Verification items for the finished model (mm, model axes). A direction names the side the tool comes from. Round coordinates to 2 decimals unless told otherwise and drop trailing zeros. Write each loop counter-clockwise with the first axis right and the second up, starting at its lowest first coordinate (ties: lowest second). Pieces come first, ordered by that corner, then holes. Notation, with made-up numbers: M 69.5,-14 L 114.5,-14 A3 cw 114.5,-9 Z; hole C -29,-22 d7. An arc over 180 degrees is marked long. Use a Markdown table: item, result. Add a question column.
from build123d import *

# Parameters (mm, degrees)
F0_W     = 58
F0_H     = 137.16
F0_R     = 1.524
F1_DEPTH = 1.27
F2_START = 1.27
F2_DEPTH = 24.13


with BuildPart() as f1:
    # F0 (on Top) → F1 (new body)
    with BuildSketch(Plane.XY):
        with Locations((0, -52.8447)):
            Rectangle(F0_W, F0_H)
        with BuildLine():
            Line((-29, 15.7353), (29, 15.7353))
            Line((29, 15.7353), (29, 21.4803))
            ThreePointArc((29, 21.4803), (28.0700640303, 23.7253640303), (25.825, 24.6553))
            Line((25.825, 24.6553), (-25.825, 24.6553))
            ThreePointArc((-25.825, 24.6553), (-28.0700640303, 23.7253640303), (-29, 21.4803))
            Line((-29, 21.4803), (-29, 15.7353))
        make_face()
        with Locations((-26.1366, 21.7678)):
            Circle(F0_R, mode=Mode.SUBTRACT)
        with Locations((26.1366, 21.7678)):
            Circle(F0_R, mode=Mode.SUBTRACT)
        with BuildLine():
            Line((-25.825, -130.3447), (25.825, -130.3447))
            ThreePointArc((25.825, -130.3447), (28.0700640303, -129.4147640303), (29, -127.1697))
            Line((29, -127.1697), (29, -121.4247))
            Line((29, -121.4247), (-29, -121.4247))
            Line((-29, -121.4247), (-29, -127.1697))
            ThreePointArc((-29, -127.1697), (-28.0700640303, -129.4147640303), (-25.825, -130.3447))
        make_face()
        with Locations((-26.1366, -127.4572)):
            Circle(F0_R, mode=Mode.SUBTRACT)
        with Locations((26.1366, -127.4572)):
            Circle(F0_R, mode=Mode.SUBTRACT)
    extrude(amount=F1_DEPTH)

    # F0 (on Top) → F2 (join)
    with BuildSketch(Plane.XY.offset(F2_START)):
        with Locations((0, -52.8447)):
            Rectangle(F0_W, F0_H)
    extrude(amount=F2_DEPTH)

    # F3 (on Right) → F4 (revolve)
    with BuildSketch(Plane.YZ):
        Polygon((5.8928, 70.612), (3.4461211403, 70.612), (2, 68.199), (0, 68.199), (0, 25.4), (14.2875, 25.4), (14.2875, 53.2638), (5.8928, 69.85), align=None)
    revolve(axis=Axis((0, 0, 43.7137000263), (0, 0, 1)))


solid = f1.part
1. Release check for a two-part mould opening along Y. For faces 4 (the flat face through (0, 0, 68.199)), 5 (the cylindrical face through (-0.628, -14.274, 39.527)), 6 (the flat face through (0, -52, 0)), 7 (the cylindrical face through (-28.045, 23.75, 0.626)) record: +Y half, -Y half, draft (parallel to the pull), parting line (faces both ways), or undercut.
2. Cross-section at C-C on z = 18. Enter the section's corners in (x, y).
3. Scan lines: line 1 along Z through (x, y) = (17.5, -103); line 2 along Y through (x, z) = (1, 46.5); line 3 along Y through (x, z) = (3, 7). Record each from-to range of solid material in increasing order. Write a range as from..to.
4. Access from +Z, -Z, +X, -X, +Y, -Y to the whole of each face (thin tool, end or side, straight path). Record for faces 1 (the flat face through (0, 15.735, 13)), 2 (the cylindrical face through (-1.77, 5.62, 70.24)), 3 (the flat face through (0, -126, 1.27)).
5. Cross-section at D-D on x = 0. Enter the section's corners in (y, z).
6. Cross-section at B-B on y = 0. Enter the section's corners in (x, z), plus the area to 3 significant figures.
7. Cross-section at A-A on x = 17. Enter the section's corners in (y, z), plus the area to 3 significant figures.
8. Depth check by flat-ended pin: pin 1 Ø4.5 at (x, y) = (7.5, 19) entering from +Z; pin 2 Ø8 at (x, z) = (-4.5, 53.5) entering from -Y; pin 3 Ø7 at (x, z) = (6.5, 9) entering from +Y. Enter the tip coordinate at first touch or a pass-through.
Answer:
| question | item | result |
|---|---|---|
| 1 | face 4 | undercut |
| 1 | face 5 | parting line |
| 1 | face 6 | draft |
| 1 | face 7 | +Y half |
| 2 | outline | M -29,-121.42 L 29,-121.42 L 29,15.74 L -29,15.74 Z |
| 3 | line 1 | z = 0..25.4 |
| 3 | line 2 | y = -14.25..14.25 |
| 3 | line 3 | y = -121.42..15.74 |
| 4 | face 1 | +Z, +X, -X, +Y |
| 4 | face 2 | +Z |
| 4 | face 3 | +Z, +X, -X, -Y |
| 5 | outline | M -130.34,0 L 24.66,0 L 24.66,1.27 L 15.74,1.27 L 15.74,25.4 L 14.29,25.4 L 14.29,53.26 L 5.89,69.85 L 5.89,70.61 L 3.45,70.61 L 2,68.2 L -2,68.2 L -3.45,70.61 L -5.89,70.61 L -5.89,69.85 L -14.29,53.26 L -14.29,25.4 L -121.42,25.4 L -121.42,1.27 L -130.34,1.27 Z |
| 6 | outline | M -29,0 L 29,0 L 29,25.4 L 14.29,25.4 L 14.29,53.26 L 5.89,69.85 L 5.89,70.61 L 3.45,70.61 L 2,68.2 L -2,68.2 L -3.45,70.61 L -5.89,70.61 L -5.89,69.85 L -14.29,53.26 L -14.29,25.4 L -29,25.4 Z |
| 6 | area | 2,600 mm^2 |
| 7 | outline | M -130.34,0 L 24.66,0 L 24.66,1.27 L 15.74,1.27 L 15.74,25.4 L -121.42,25.4 L -121.42,1.27 L -130.34,1.27 Z |
| 7 | area | 3,510 mm^2 |
| 8 | pin 1 | stops at z = 1.27 |
| 8 | pin 2 | stops at y = -14.28 |
| 8 | pin 3 | stops at y = 15.74 |
